Work out the finished part from the listing and answer in its coordinate system (mm). Face numbers are marked on the shaded views. A direction names the side the tool comes from. Coordinates: 2 decimals unless noted, no trailing zeros. Loops run counter-clockwise (first coordinate to the right, second up) from the corner with the lowest first, then second, coordinate; pieces in that order, holes last. Notation, with made-up numbers: (81.25, -1) -> (101.25, -1) arc R13 ccw to (101.25, 4) -> close; hole circle Ø6 at (6.25, -33). An arc over 180 degrees is marked (long way). Answer as CSV lines item,"result".
```python
from build123d import *

# Parameters (mm, degrees)
F0_W     = 457.2
F0_H     = 215.9
F1_DEPTH = 19.05
F2_W     = 50.8
F2_H     = 203.2
F2_W_2   = 15.875
F2_H_2   = 88.9
F2_W_3   = 19.05
F2_H_3   = 152.4
F2_W_4   = 57.15
F2_W_5   = 25.4
F2_H_4   = 177.8
F2_W_6   = 28.575
F2_H_5   = 180.975
F2_R     = 14.2875
F2_R_2   = 11.1125
F2_R_3   = 9.525
F3_DEPTH = 7.62
F5_DEPTH = 7.62


# Not quite as in the source:
# - a length typed as a fraction of an inch, garbled in the dataset ("3 / 203.2 mm" for 3/8 in), is restored


with BuildPart() as f1:
    # F0 (on Front) → F1 (new body)
    with BuildSketch(Plane.XZ):
        with Locations((34.5792232292, 7.7549852431)):
            Rectangle(F0_W, F0_H)
    extrude(amount=F1_DEPTH)

    # F2 (on face) → F3 (cut)
    with BuildSketch(Plane.XZ.offset(19.05)):
        with Locations((-163.2603832245, 5.173290801)):
            Rectangle(F2_W, F2_H)
        with Locations((-108.1939504743, -22.3739650816)):
            Rectangle(F2_W_2, F2_H_2)
        with Locations((-36.7521092981, 31.5419817448)):
            Rectangle(F2_W_3, F2_H_3)
        with Locations((32.6018253148, 6.1419817448)):
            Rectangle(F2_W_4, F2_H)
        with Locations((108.8770244598, 5.1134674311)):
            Rectangle(F2_W_5, F2_H_4)
        with Locations((165.9826848984, 5.1134674311)):
            Rectangle(F2_W_5, F2_H_4)
        with Locations((231.9335953236, 4.6242426157)):
            Rectangle(F2_W_6, F2_H_5)
        with Locations((-116.1314504743, 96.762670864)):
            Circle(F2_R)
        with Locations((-83.2345709205, 95.660790801)):
            Circle(F2_R_2)
        with Locations((-83.7836638093, 57.2242997587)):
            Circle(F2_R_3)
        with Locations((-120.1787297428, 57.6790883665)):
            Circle(F2_R_3)
    extrude(amount=-F3_DEPTH, mode=Mode.SUBTRACT)

    # F4 (on face) → F5 (cut)
    with BuildSketch(Plane.XZ.offset(19.05)):
        with BuildLine():
            ThreePointArc((-100.2564504743, -31.8989650816), (-93.5212583835, -29.1091571724), (-90.7314504743, -22.3739650816))
            ThreePointArc((-90.7314504743, -22.3739650816), (-93.5212583835, -15.6387729908), (-100.2564504743, -12.8489650816))
            Line((-100.2564504743, -12.8489650816), (-100.2564504743, -31.8989650816))
        make_face()
        with BuildLine():
            ThreePointArc((-27.2271092981, 2.0650514647), (-20.4919172073, 4.8548593739), (-17.7021092981, 11.5900514647))
            ThreePointArc((-17.7021092981, 11.5900514647), (-20.4919172073, 18.3252435555), (-27.2271092981, 21.1150514647))
            Line((-27.2271092981, 21.1150514647), (-27.2271092981, 2.0650514647))
        make_face()
        with BuildLine():
            ThreePointArc((121.5770244598, -4.4115325689), (128.3122165506, -1.6217246597), (131.1020244598, 5.1134674311))
            ThreePointArc((131.1020244598, 5.1134674311), (128.3122165506, 11.8486595219), (121.5770244598, 14.6384674311))
            Line((121.5770244598, 14.6384674311), (121.5770244598, -4.4115325689))
        make_face()
        with BuildLine():
            ThreePointArc((178.6826848984, -4.4115325689), (185.4178769892, -1.6217246597), (188.2076848984, 5.1134674311))
            ThreePointArc((188.2076848984, 5.1134674311), (185.4178769892, 11.8486595219), (178.6826848984, 14.6384674311))
            Line((178.6826848984, 14.6384674311), (178.6826848984, -4.4115325689))
        make_face()
        with BuildLine():
            ThreePointArc((217.6460953236, -4.9007573843), (224.3812874144, -2.1109494751), (227.1710953236, 4.6242426157))
            ThreePointArc((227.1710953236, 4.6242426157), (224.3812874144, 11.3594347065), (217.6460953236, 14.1492426157))
            Line((217.6460953236, 14.1492426157), (217.6460953236, -4.9007573843))
        make_face()
        with BuildLine():
            Line((217.6460953236, -4.9007573843), (217.6460953236, 14.1492426157))
            ThreePointArc((217.6460953236, 14.1492426157), (208.1210953236, 4.6242426157), (217.6460953236, -4.9007573843))
        make_face()
    extrude(amount=-F5_DEPTH, mode=Mode.SUBTRACT)


solid = f1.part
```
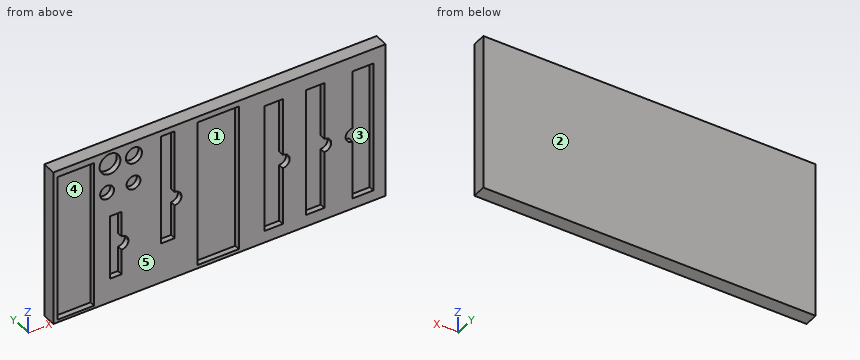
(1) A cutting plane is placed at A-A, the plane z = 77. Write down the section's boundary in (x, y), and give its area (3 significant figures).
Computed values:
outline,"(-194.02, -19.05) -> (-188.66, -19.05) -> (-188.66, -11.43) -> (-137.86, -11.43) -> (-137.86, -19.05) -> (-46.28, -19.05) -> (-46.28, -11.43) -> (-27.23, -11.43) -> (-27.23, -19.05) -> (4.03, -19.05) -> (4.03, -11.43) -> (61.18, -11.43) -> (61.18, -19.05) -> (96.18, -19.05) -> (96.18, -11.43) -> (121.58, -11.43) -> (121.58, -19.05) -> (153.28, -19.05) -> (153.28, -11.43) -> (178.68, -11.43) -> (178.68, -19.05) -> (217.65, -19.05) -> (217.65, -11.43) -> (246.22, -11.43) -> (246.22, -19.05) -> (263.18, -19.05) -> (263.18, 0) -> (-194.02, 0) -> close"
area,"7,140 mm2"
(2) A cutting plane is placed at B-B, the plane z = -52.5. Write down the section's boundary in (x, y), and give its area (3 significant figures).
Computed values:
outline,"(-194.02, -19.05) -> (-188.66, -19.05) -> (-188.66, -11.43) -> (-137.86, -11.43) -> (-137.86, -19.05) -> (-116.13, -19.05) -> (-116.13, -11.43) -> (-100.26, -11.43) -> (-100.26, -19.05) -> (4.03, -19.05) -> (4.03, -11.43) -> (61.18, -11.43) -> (61.18, -19.05) -> (96.18, -19.05) -> (96.18, -11.43) -> (121.58, -11.43) -> (121.58, -19.05) -> (153.28, -19.05) -> (153.28, -11.43) -> (178.68, -11.43) -> (178.68, -19.05) -> (217.65, -19.05) -> (217.65, -11.43) -> (246.22, -11.43) -> (246.22, -19.05) -> (263.18, -19.05) -> (263.18, 0) -> (-194.02, 0) -> close"
area,"7,160 mm2"
(3) Which of the six approach directions +Z, -Z, +X, -X, +Y, -Y give full straight-line access (tool end or side, diameter ignored) to the marked faces 1 and 2?
Computed values:
face 1,"-Y"
face 2,"+Z, -Z, +X, -X, +Y"
(4) Consider line 1 along Z through (x, y) = (237.5, -17.75); line 2 along Z through (x, y) = (-46, -14.5); line 3 along Y through (x, z) = (120, -6.5). Determine where each line is inside the solid, lowest interval first.
Computed values:
line 1,"-100.2 to -85.86, 95.11 to 115.7"
line 2,"-100.2 to -44.66, 107.74 to 115.7"
line 3,"-11.43 to 0"
(5) For a pull along X with two mould halves and no side action, classify the marked faces 3, 4 and 5 as pulls with the +X half, pulls with the -X half, needs draft (parallel to the pull), parting line crosses it, or undercut.
Computed values:
face 3,"undercut"
face 4,"undercut"
face 5,"needs draft"
